Design review of the part built by this model. Coordinates are the model's own, in mm. A direction names the side the tool comes from. Coordinates: 2 decimals unless noted, no trailing zeros. Write each loop counter-clockwise with the first axis right and the second up, starting at its lowest first coordinate (ties: lowest second). Pieces come first, ordered by that corner, then holes. Notation, with made-up numbers: (48.5, -20.75) - (98.5, -20.75) arc R19 ccw to (98.5, 6.25) - close; hole circle Ø1 at (-32.5, -28.5). An arc over 180 degrees is marked (long way). Use a Markdown table: item, result.
from build123d import *

# Parameters (mm, degrees)
CYLINDER008_R      = 1.65
CYLINDER008_DEPTH  = 10
CYLINDER009_R      = 3.2
CYLINDER009_DEPTH  = 10
CYLINDER007_R      = 2
CYLINDER007_DEPTH  = 10
CYLINDER006_R      = 1.65
CYLINDER006_DEPTH  = 50
BOX014_W           = 5
BOX014_H           = 3
BOX014_DEPTH       = 30
BOX012_W           = 19.5
BOX012_H           = 21
BOX012_DEPTH       = 30
BOX011_W           = 59
BOX011_H           = 5
BOX011_DEPTH       = 30
FILLET001_R        = 5
FILLET002_R        = 7
CHAMFER006004_SIZE = 5
CHAMFER006005_SIZE = 5
CHAMFER006006_SIZE = 0.4


with BuildPart() as cylinder008:
    # Cylinder008 → Cylinder008 (new body)
    with BuildSketch(Plane(origin=(37.5, 0, 23.5), x_dir=(1, 0, 0), z_dir=(0, -1, 0))):
        Circle(CYLINDER008_R)
    extrude(amount=CYLINDER008_DEPTH)


with BuildPart() as fusion004:
    # Cylinder009 → Cylinder009 (new body)
    with BuildSketch(Plane(origin=(37.5, -7, 23.5), x_dir=(1, 0, 0), z_dir=(0, -1, 0))):
        Circle(CYLINDER009_R)
    extrude(amount=CYLINDER009_DEPTH)

    # Fusion004: union Cylinder008
    add(cylinder008.part)


with BuildPart() as cylinder007:
    # Cylinder007 → Cylinder007 (new body)
    with BuildSketch(Plane(origin=(15, 0, 23.5), x_dir=(1, 0, 0), z_dir=(0, -1, 0))):
        Circle(CYLINDER007_R)
    extrude(amount=CYLINDER007_DEPTH)


with BuildPart() as cylinder006:
    # Cylinder006 → Cylinder006 (new body)
    with BuildSketch(Plane(origin=(-14, 6.5, -4), x_dir=(1, 0, 0), z_dir=(0, 0, 1))):
        Circle(CYLINDER006_R)
    extrude(amount=CYLINDER006_DEPTH)


with BuildPart() as cube013:
    # Box014 → Box014 (new body)
    with BuildSketch(Plane(origin=(-0.5, -4, 8.5), x_dir=(1, 0, 0), z_dir=(0, 0, 1))):
        with Locations((2.5, 1.5)):
            Rectangle(BOX014_W, BOX014_H)
    extrude(amount=BOX014_DEPTH)


with BuildPart() as cube012:
    # Box012 → Box012 (new body)
    with BuildSketch(Plane(origin=(-20, -9, 8.5), x_dir=(1, 0, 0), z_dir=(0, 0, 1))):
        with Locations((9.75, 10.5)):
            Rectangle(BOX012_W, BOX012_H)
    extrude(amount=BOX012_DEPTH)


with BuildPart() as chamfer006006:
    # Box011 → Box011 (new body)
    with BuildSketch(Plane(origin=(-14, -9, 8.5), x_dir=(1, 0, 0), z_dir=(0, 0, 1))):
        with Locations((29.5, 2.5)):
            Rectangle(BOX011_W, BOX011_H)
    extrude(amount=BOX011_DEPTH)

    # Fusion003: union Cube013, Cube012
    add(cube013.part)
    add(cube012.part)

    # Cut010011008009003016026008003006: cut Cylinder006
    add(cylinder006.part, mode=Mode.SUBTRACT)

    # Fillet001
    fillet001_edges = [chamfer006006.edges().sort_by_distance(p)[0] for p in [
        (-20, 12, 23.5),
    ]]
    fillet(fillet001_edges, radius=FILLET001_R)

    # Fillet002
    fillet002_edges = [chamfer006006.edges().sort_by_distance(p)[0] for p in [
        (-0.5, 12, 23.5),
    ]]
    fillet(fillet002_edges, radius=FILLET002_R)

    # Chamfer006004
    chamfer006004_edges = [chamfer006006.edges().sort_by_distance(p)[0] for p in [
        (-20, -9, 23.5),
    ]]
    chamfer(chamfer006004_edges, length=CHAMFER006004_SIZE)

    # Chamfer006005
    chamfer006005_edges = [chamfer006006.edges().sort_by_distance(p)[0] for p in [
        (45, -6.5, 8.5),
        (45, -6.5, 38.5),
    ]]
    chamfer(chamfer006005_edges, length=CHAMFER006005_SIZE)

    # Cut010011008009003016026008003007: cut Cylinder007
    add(cylinder007.part, mode=Mode.SUBTRACT)

    # Cut010011008009003016026008003008: cut Fusion004
    add(fusion004.part, mode=Mode.SUBTRACT)

    # Chamfer006006
    chamfer006006_edges = [chamfer006006.edges().sort_by_distance(p)[0] for p in [
        (34.3, -9, 23.5),
        (22.25, -4, 8.5),
        (42.5, -4, 11),
        (45, -4, 23.5),
        (22.25, -4, 38.5),
        (42.5, -4, 36),
        (42.5, -9, 11),
        (40, -6.5, 8.5),
        (4.5, -2.5, 38.5),
        (4.5, -2.5, 8.5),
        (45, -9, 23.5),
        (42.5, -9, 36),
        (13, -9, 23.5),
        (2, -1, 8.5),
        (2, -1, 38.5),
        (-0.5, 2, 38.5),
        (-0.5, 2, 8.5),
        (-2.550253, 9.949747, 8.5),
        (-2.550253, 9.949747, 38.5),
        (-11.25, 12, 8.5),
        (-11.25, 12, 38.5),
        (-18.535534, 10.535534, 8.5),
        (-18.535534, 10.535534, 38.5),
        (-20, 1.5, 38.5),
        (-20, 1.5, 8.5),
        (-17.5, -6.5, 8.5),
        (-17.5, -6.5, 38.5),
        (12.5, -9, 8.5),
        (-15.65, 6.5, 8.5),
        (-15.65, 6.5, 38.5),
        (12.5, -9, 38.5),
    ]]
    chamfer(chamfer006006_edges, length=CHAMFER006006_SIZE)


solid = chamfer006006.part
(1) Take a section at B-B on x = 37.5. Write out the cut boundary in (y, z).
Determined:
| item | result |
|---|---|
| outline | (-9, 8.9) - (-8.6, 8.5) - (-4.4, 8.5) - (-4, 8.9) - (-4, 21.85) - (-7, 21.85) - (-7, 20.3) - (-8.6, 20.3) - (-9, 19.9) - close; (-9, 27.1) - (-8.6, 26.7) - (-7, 26.7) - (-7, 25.15) - (-4, 25.15) - (-4, 38.1) - (-4.4, 38.5) - (-8.6, 38.5) - (-9, 38.1) - close |
(2) Take a section at D-D on x = 3. Write out the cut boundary in (y, z), and give its area (3 significant figures).
Determined:
| item | result |
|---|---|
| outline | (-9, 8.9) - (-8.6, 8.5) - (-1.4, 8.5) - (-1, 8.9) - (-1, 38.1) - (-1.4, 38.5) - (-8.6, 38.5) - (-9, 38.1) - close |
| area | 240 mm2 |
(3) Draft analysis for pull direction X (two halves, no side actions). For faces 3 (the flat face through (-17.396, -6.326, 8.703)), 4 (the cylindrical face through (-12.476, 5.868, 23.296)), 5 (the flat face through (24, -4, 23)), 6 (the flat face through (42.47, -8.8, 11.25)), state which applies: +X half, -X half, draft (parallel to the pull), parting line (faces both ways), or undercut.
Determined:
| item | result |
|---|---|
| face 3 | -X half |
| face 4 | undercut |
| face 5 | draft |
| face 6 | +X half |
(4) Take a section at A-A on z = 23.5. State how many separate pieces and enclosed holes the cut face has, and give its area (3 significant figures).
Determined:
| item | result |
|---|---|
| separate pieces | 3 |
| enclosed holes | 1 |
| area | 572 mm2 |
(5) Take a section at C-C on z = 31.5. Write out the cut boundary in (x, y).
Determined:
| item | result |
|---|---|
| outline | (-20, -4) - (-15, -9) - (44.6, -9) - (45, -8.6) - (45, -4.4) - (44.6, -4) - (4.5, -4) - (4.5, -1) - (-0.5, -1) - (-0.5, 5) arc R7 ccw to (-7.5, 12) - (-15, 12) arc R5 ccw to (-20, 7) - close; hole circle Ø3.3 at (-14, 6.5) |
(6) For L1, parallel to Z at x = 15, y = -6.8; L2, parallel to Y at x = -14, z = 20; L3, parallel to X at y = -7.8, z = 23.5, list the stretches that pass through material, from the lowest coordinate up. Write a range as from..to.
Determined:
| item | result |
|---|---|
| L1 | 8.5..21.5, 25.5..38.5 |
| L2 | -9..4.85, 8.15..12 |
| L3 | -16.2..13, 17..34.3, 40.7..45 |
(7) For pin 1 (1.5 mm diameter, centred on y = -2.5, z = 25, fed in from +X); pin 2 (10 mm diameter, centred on y = 5, z = 13.5, fed in from +X); pin 3 (5 mm diameter, centred on x = 37.5, z = 23.5, fed in from -Y), all flat-tipped, find the tip position at first contact; note any pin that passes through.
Determined:
| item | result |
|---|---|
| pin 1 | x = 4.5 |
| pin 2 | x = -0.5 |
| pin 3 | y = -7 |
(8) Machinability: for faces 1 (the conical face through (-18.296, 10.37, 8.614)), 2 (the flat face through (39, -7, 22)), which of the approach directions +Z, -Z, +X, -X, +Y, -Y give a long, thin tool a straight path to every point of the face, cutting with its end or side? Answer none if there is none.
Determined:
| item | result |
|---|---|
| face 1 | -Z, -X, +Y |
| face 2 | -Y |
